from build123d import *

# Parameters (mm, degrees)
SKETCH1_W           = 400
SKETCH1_H           = 300
BOSS_EXTRUDE1_DEPTH = 5
SKETCH2_W           = 400
SKETCH2_H           = 300
SKETCH2_W_2         = 394
SKETCH2_H_2         = 294
BOSS_EXTRUDE2_DEPTH = 165
SKETCH3_W           = 350
SKETCH3_H           = 240
BOSS_EXTRUDE3_DEPTH = 26


with BuildPart() as part:
    # Sketch1 → Boss-Extrude1 (new body)
    with BuildSketch(Plane.XY):
        Rectangle(SKETCH1_W, SKETCH1_H)
    extrude(amount=BOSS_EXTRUDE1_DEPTH)

    # Sketch2 → Boss-Extrude2 (add)
    with BuildSketch(Plane.XY):
        Rectangle(SKETCH2_W, SKETCH2_H)
        Rectangle(SKETCH2_W_2, SKETCH2_H_2, mode=Mode.SUBTRACT)
    extrude(amount=BOSS_EXTRUDE2_DEPTH)

    # Sketch3 → Boss-Extrude3 (add)
    with BuildSketch(Plane.XY):
        Rectangle(SKETCH3_W, SKETCH3_H)
    extrude(amount=BOSS_EXTRUDE3_DEPTH)


solid = part.part
The listing builds one solid part. Answer for the finished solid, in the listing's coordinates (mm). A direction names the side the tool comes from. Coordinates: 2 decimals unless noted, no trailing zeros. Write each loop counter-clockwise with the first axis right and the second up, starting at its lowest first coordinate (ties: lowest second). Pieces come first, ordered by that corner, then holes. Notation, with made-up numbers: (-7, -29) - (37, -29) arc R11 cw to (37, -9) - close; hole circle Ø4 at (73, 68.25). An arc over 180 degrees is marked (long way). Put each result on its own line as item: value.
1. The part is cut by section A-A on z = 93.5. Give the vertices of the cut face in (x, y), plus the area to 3 significant figures.
Answer sheet:
outline: (-200, -150) - (200, -150) - (200, 150) - (-200, 150) - close; hole (-197, -147) - (197, -147) - (197, 147) - (-197, 147) - close
area: 4,160 mm^2
2. The part is cut by section C-C on x = -144. Give the vertices of the cut face in (y, z), plus the area to 3 significant figures.
Answer sheet:
outline: (-150, 0) - (150, 0) - (150, 165) - (147, 165) - (147, 5) - (120, 5) - (120, 26) - (-120, 26) - (-120, 5) - (-147, 5) - (-147, 165) - (-150, 165) - close
area: 7,500 mm^2
3. The part is cut by section B-B on y = -76. Give the vertices of the cut face in (x, z).
Answer sheet:
outline: (-200, 0) - (200, 0) - (200, 165) - (197, 165) - (197, 5) - (175, 5) - (175, 26) - (-175, 26) - (-175, 5) - (-197, 5) - (-197, 165) - (-200, 165) - close
4. Determine the mould class of faces 1 (the face through (-2, 2, 26)), 2 (the face through (-3, -150, 81)), 3 (the face through (200, -2, 81)) for opening direction X: pulls with the +X half, pulls with the -X half, needs draft (parallel to the pull), parting line crosses it, or undercut.
Answer sheet:
face 1: undercut
face 2: needs draft
face 3: pulls with the +X half
5. Flat-ended cylindrical pins translate along their axes: pin 1 Ø6 at (x, y) = (128, 43.5) entering from +Z; pin 2 Ø1.5 at (x, y) = (149.5, -41.5) entering from -Z. Find the tip coordinate at first contact, or state that the pin passes through.
Answer sheet:
pin 1: stops at z = 26
pin 2: stops at z = 0
6. Find the intervals of material crossed by line 1 along X through (y, z) = (42, 10); line 2 along Y through (x, z) = (90.5, 148); line 3 along X through (y, z) = (-21.5, 52), in increasing order. Write a range as from..to.
Answer sheet:
line 1: x = -200..-197, -175..175, 197..200
line 2: y = -150..-147, 147..150
line 3: x = -200..-197, 197..200
7. A tool of negligible diameter and unlimited length cuts with its end or side. For faces 4 (the face through (-200, -2, 81)), 5 (the face through (-3, 147, 84)), from which of +Z, -Z, +X, -X, +Y, -Y can it reach the whole face along a straight path? Write none if from no direction.
Answer sheet:
face 4: +Z, -Z, -X, +Y, -Y
face 5: +Z
